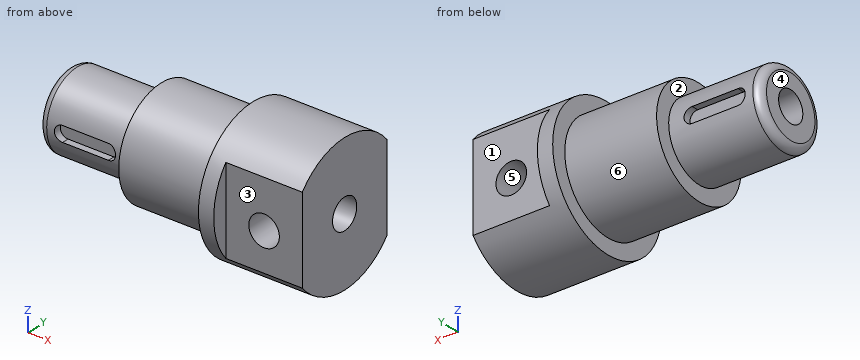
Autodesk Inventor part; units mm, degrees
ref_plane "Plano de trabajo1" through (0, 10, 0) normal (0, 1, 0) x (-1, 0, 0)
ref_plane "YZ Plane" through (0, 0, 0) normal (1, 0, 0) x (0, 1, 0)
ref_plane "XY Plane" through (0, 0, 0) normal (0, 0, 1) x (1, 0, 0)
sketch "Boceto1" plane through (0, 0, 0) normal (0, 1, 0) x (-1, 0, 0)
  line L0 (0, 0) -> (72, 0)
  line L1 (72, 0) -> (72, 10)
  line L2 (72, 10) -> (48, 10)
  line L3 (48, 10) -> (48, 14)
  line L4 (48, 14) -> (24, 14)
  line L5 (24, 14) -> (24, 18)
  line L6 (24, 18) -> (0, 18)
  line L7 (0, 18) -> (0, 0)
  dimension "d15" = 72
  dimension "d16" = 10
  dimension "d17" = 24
  dimension "d18" = 4
  dimension "d19" = 24
  dimension "d20" = 4
revolve "Revolución2" add sketch "Boceto1" angle 360 about axis through (0, 0, 0) along (-1, 0, 0)
sketch "Boceto2" plane through (0, 0, 0) normal (1, 0, 0) x (0, 0, -1)
  line L0 (-11.3137, 14) -> (11.3137, 14)
  circle A0 centre (0, 0) radius 18
  line L1 (-11.3137, -14) -> (11.3137, -14)
  dimension "d22" = 14
  dimension "d25" = 14
extrude "Extrusión1" cut sketch "Boceto2" against normal blind 20 contours A0 L0 | L1 A0
sketch "Boceto3" plane through (0, 14, 11.3137) normal (0, 1, 0) x (1, 0, 0)
  circle A0 centre (-10, 12.6274) radius 4
  line L0 (-20, 22.6274) -> (0, 22.6274)
  line L1 (0, 22.6274) -> (0, 0)
  point P0 (0, 11.3137)
  dimension "d26" = 8
  dimension "d28" = 10
  dimension "d29" = 10
extrude "Extrusión2" cut sketch "Boceto3" against normal through all
sketch "Boceto4" plane through (0, 0, 0) normal (1, 0, 0) x (0, 0, -1)
  circle A0 centre (0, 0) radius 4
  dimension "d32" = 8
extrude "Extrusión3" cut sketch "Boceto4" against normal through all
fillet "Empalme1" radius 2 1 edges at (-72, 0, -10)
ref_plane "Plano de trabajo1" through (0, 10, 0) normal (0, 1, 0) x (-1, 0, 0)
sketch "Boceto5" plane through (0, 10, 0) normal (0, 1, 0) x (-1, 0, 0)
  line L0 (54, 2) -> (66, 2)
  line L1 (68, 0) -> (68, 0)
  line L2 (66, -2) -> (54, -2)
  line L3 (52, 0) -> (52, 0)
  line L4 (52, 2) -> (68, -2) construction
  line L5 (68, 2) -> (52, -2) construction
  arc A0 (68, 0) -> (66, 2) centre (66, 0) ccw
  arc A1 (66, -2) -> (68, 0) centre (66, 0) ccw
  arc A2 (54, 2) -> (52, 0) centre (54, 0) ccw
  arc A3 (52, 0) -> (54, -2) centre (54, 0) ccw
  line L6 (48, -14) -> (48, 14)
  point P0 (0, 0)
  point P1 (60, 0)
  point P2 (52, 0)
  point P3 (68, 0)
  dimension "d37" = 16
  dimension "d38" = 4
  dimension "d39" = 2
  dimension "d40" = 12
extrude "Extrusión4" cut sketch "Boceto5" against normal blind 2
mirror "Simetría1" about plane through (0, 0, 0) normal (0, 1, 0) of "Extrusión4"
properties part number "Pieza de practica 11"
CAD build for the part. Positions are in the model's coordinates, mm. Face numbers are marked on the shaded views. A direction names the side the tool comes from. Coordinates: 2 decimals unless noted, no trailing zeros. Order: outer loops, then holes, each group sorted by start corner. A loop starts at its lowest first (then second) coordinate and runs counter-clockwise, first axis right, second up.
(1) Saw through at C-C, the plane x = -60. Write the cut outline in (y, z).
Solution:
outline: (-9.8, -2) arc R10 ccw to (9.8, -2) - (8, -2) - (8, 2) - (9.8, 2) arc R10 ccw to (-9.8, 2) - (-8, 2) - (-8, -2) - close; hole circle Ø8 at (0, 0)
(2) Saw through at A-A, the plane y = 0. Write the cut outline in (x, z), and give its area (3 significant figures).
Solution:
outline: (-72, -8) arc R2 ccw to (-70, -10) - (-48, -10) - (-48, -14) - (-24, -14) - (-24, -18) - (0, -18) - (0, -4) - (-7.04, -4) arc R4 cw to (-12.96, -4) - (-72, -4) - close; (-72, 4) - (0, 4) - (0, 18) - (-24, 18) - (-24, 14) - (-48, 14) - (-48, 10) - (-70, 10) arc R2 ccw to (-72, 8) - close
area: 1,430 mm2
(3) Pin check, flat tips, straight feed: pin 1 Ø1.2 at (y, z) = (15.5, 1.5) entering from +X; pin 2 Ø1.4 at (x, y) = (-58.5, -9) entering from +Z; pin 3 Ø5 at (x, z) = (-19.5, 13.5) entering from +Y. Stop position of each tip, or through.
Solution:
pin 1: stops at x = -20
pin 2: stops at z = 5.58
pin 3: stops at y = 14.21
(4) Saw through at B-B, the plane x = -10. Write the cut outline in (y, z), and give its area (3 significant figures).
Solution:
outline: (-14, -11.31) arc R18 ccw to (14, -11.31) - (14, -5.31) - (-14, -5.31) - close; (-14, 2.69) - (-2.96, 2.69) arc R4 cw to (2.96, 2.69) - (14, 2.69) - (14, 11.31) arc R18 ccw to (-14, 11.31) - close
area: 665 mm2
(5) Which spindle directions (+Z, -Z, +X, -X, +Y, -Y) get a long thin tool onto all of the face, cutting with end or side? Do the marked faces 1, 2 and 3. Say none if no direction does.
Solution:
face 1: +Z, -Z, +X, +Y
face 2: -X
face 3: +Z, -Z, +X, -Y
(6) Saw through at D-D, the plane y = -12.5. Write the cut outline in (x, z).
Solution:
outline: (-48, -6.3) - (-24, -6.3) - (-24, -12.95) - (0, -12.95) - (0, 12.95) - (-24, 12.95) - (-24, 6.3) - (-48, 6.3) - close; hole circle Ø8 at (-10, -1.31)
(7) Mould opens along X. For the marked faces 4, 5 and 6 say: released by +X, released by -X, zero draft, split by the parting line, or undercut.
Solution:
face 4: released by -X
face 5: undercut
face 6: zero draft
(8) Drill centre lines: L1, parallel to Y at x = -3, z = 0; L2, parallel to X at y = 10, z = 8; L3, parallel to Y at x = -56, z = 0. Where is each one in solid material? Low to high.
Solution:
L1: y = -14 to -4, 4 to 14
L2: x = -48 to 0
L3: y = -8 to -4, 4 to 8
